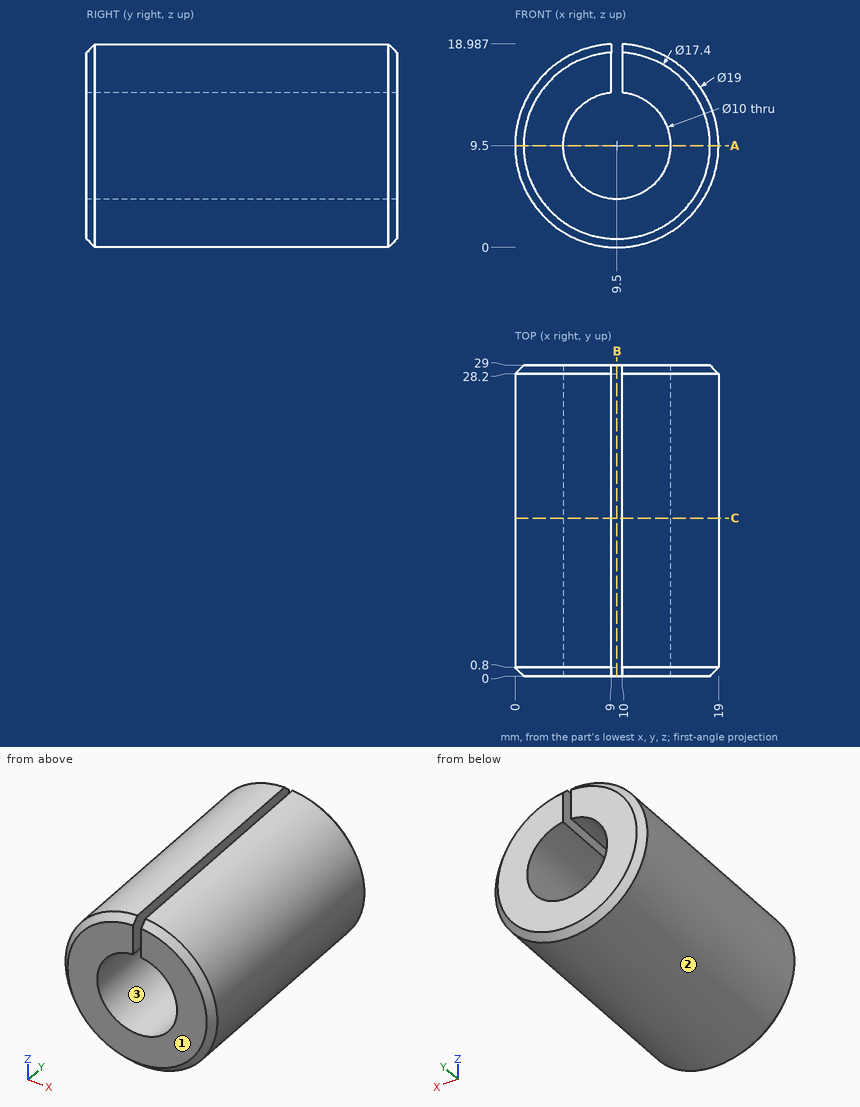
Drawing for the job (mm, zero at the part's lowest x, y, z). Coordinates: 2 decimals unless noted, no trailing zeros. Order: outer loops, then holes, each group sorted by start corner. A loop starts at its lowest first (then second) coordinate and runs counter-clockwise, first axis right, second up. Notation, with made-up numbers: (88.25, 44.5) - (100.25, 44.5) arc R12 ccw to (100.25, 54.5) - close; hole circle Ø10 at (-5.5, 21.25). An arc over 180 degrees is marked (long way). Use a Markdown table: item, result. Add a question column.
(1) Drill centre lines: line 1 along X through (y, z) = (19.5, 9.5); line 2 along Z through (x, y) = (12.25, 26); line 3 along X through (y, z) = (2.5, 14.75). Where is each one in solid material? Low to high. Write a range as [from, to].
(2) Pull direction Z, two halves, no side cores. Call the marked faces 1, 2 and 3: +Z half, -Z half, draft (parallel to the pull), parting line (faces both ways), or undercut.
(3) Saw through at B-B (x = 9.5). Give the cut face in (y, z), then the cut area to 3 significant figures.
(4) Saw through at C-C (y = 14.75). Give the cut face in (x, z) (1 decimal), then the cut area to 4 significant figures.
(5) Saw through at A-A (z = 9.5). Give the cut face in (x, y), then the cut area to 3 significant figures.
(6) Flat gauge pins, fed straight in: pin 1 (2 mm diameter, centred on x = 10.5, z = 6, fed in from -Y); pin 2 (1.5 mm diameter, centred on y = 6.5, z = 2.5, fed in from +X) (1 decimal); pin 3 (5 mm diameter, centred on y = 19, z = 17, fed in from +X); pin 4 (1.5 mm diameter, centred on x = 16.5, y = 19.5, fed in from -Z) (1 decimal). Where does each tip first touch, or does it go through?
Solved:
| question | item | result |
|---|---|---|
| 1 | line 1 | x = [0, 4.5], [14.5, 19] |
| 1 | line 2 | z = [0.41, 5.32], [13.68, 18.59] |
| 1 | line 3 | x = [1.58, 9], [10, 17.42] |
| 2 | face 1 | draft |
| 2 | face 2 | parting line |
| 2 | face 3 | undercut |
| 3 | outline | (0, 0.8) - (0.8, 0) - (28.2, 0) - (29, 0.8) - (29, 4.5) - (0, 4.5) - close |
| 3 | area | 130 mm² |
| 4 | outline | (9, 14.5) - (9, 19) arc R9.5 ccw (long way) to (10, 19) - (10, 14.5) arc R5 cw (long way) to start |
| 4 | area | 200.5 mm² |
| 5 | outline | (0, 0.8) - (0.8, 0) - (4.5, 0) - (4.5, 29) - (0.8, 29) - (0, 28.2) - close; (14.5, 0) - (18.2, 0) - (19, 0.8) - (19, 28.2) - (18.2, 29) - (14.5, 29) - close |
| 5 | area | 260 mm² |
| 6 | pin 1 | passes through |
| 6 | pin 2 | stops at x = 16.7 |
| 6 | pin 3 | stops at x = 17.58 |
| 6 | pin 4 | stops at z = 2.3 |
